Build history of the part. All positions in model axes, mm. A direction names the side the tool comes from. Give positions to 0.01 mm unless a question says otherwise; leave off trailing zeros. Loops run counter-clockwise (first coordinate to the right, second up) from the corner with the lowest first, then second, coordinate; pieces in that order, holes last. Notation, with made-up numbers: M 79,-9 L 126,-9 A30 cw 126,26 Z; hole C 19.5,50 d8. An arc over 180 degrees is marked long. Answer as a JSON object with one key per item and string values. Group by question number.
1. Slice it at D-D (z = 40). List the corners of the cut face in (x, y), then the cut area to 3 significant figures.
2. 3-axis set-ups, long thin cutter, end or side, ignore diameter. For faces 1 (the face through (25, 17.526, 25)), 2 (the face through (-44, 0, 0)), 3 (the face through (-43, 0, 17)): which of +Z, -Z, +X, -X, +Y, -Y reach the whole face in a straight line?
3. Slice it at C-C (x = 11.5). List the corners of the cut face in (y, z).
4. Slice it at B-B (x = 0). List the corners of the cut face in (y, z).
5. Mould opens along X. For faces 4 (the face through (35.708, 8.64, -35.446)), 5 (the face through (-1, -128.778, -1)), 6 (the face through (-57.095, 8.64, -2.513)) say: released by +X, released by -X, zero draft, split by the parting line, or undercut.
6. Slice it at A-A (z = 0). List the corners of the cut face in (x, y), then the cut area to 3 significant figures.
7. Drop flat-ended pins along their axis: pin 1 Ø7.5 at (x, z) = (46.101, 0) entering from +Y; pin 2 Ø6 at (y, z) = (-79.5, 35.5) entering from +X; pin 3 Ø10 at (x, y) = (8.5, -8) entering from -Z. Give the stop position or say it passes through.
8. Drill centre lines: line 1 along Z through (x, y) = (0, 12); line 2 along Y through (x, z) = (-22, 19); line 3 along Y through (x, z) = (23, 50). Where is each one in solid material? Low to high. Write a range as [from, to].
from build123d import *

# Parameters (mm, degrees)
SKETCH1_R           = 57.15
SKETCH1_R_2         = 30.099
EXTRUDE_THIN1_DEPTH = 17.526
SKETCH2_R           = 4.2164
CUT_EXTRUDE2_DEPTH  = 17.526
CIRPATTERN1_COUNT   = 8
SKETCH5_R           = 45.72
EXTRUDE1_DEPTH      = 128.778


with BuildPart() as part:
    # Sketch1 → Extrude-Thin1 (new body)
    with BuildSketch(Plane(origin=(0, 0, 0), x_dir=(1, 0, 0), z_dir=(0, 1, 0))):
        Circle(SKETCH1_R)
        Circle(SKETCH1_R_2, mode=Mode.SUBTRACT)
    extrude(amount=EXTRUDE_THIN1_DEPTH)

    # Sketch2 → Cut-Extrude2 (cut)
    with BuildSketch(Plane(origin=(0, 0, 0), x_dir=(1, 0, 0), z_dir=(0, 1, 0))):
        with Locations(Location((0, 46.101, 0), (0, 0, 270))):
            Circle(SKETCH2_R)
    cut_extrude2 = extrude(amount=CUT_EXTRUDE2_DEPTH, mode=Mode.SUBTRACT)

    # CirPattern1: Cut-Extrude2 ×8 about axis
    cirpattern1_axis = Axis((0, 0, 0), (0, 1, 0))
    for i in range(1, CIRPATTERN1_COUNT):
        add(cut_extrude2.rotate(cirpattern1_axis, i * 360 / CIRPATTERN1_COUNT), mode=Mode.SUBTRACT)

    # Sketch5 → Extrude1 (add)
    with BuildSketch(Plane.XZ):
        with Locations(Location((0, 0, 0), (0, 0, 95.242365855))):
            Circle(SKETCH5_R)
    extrude(amount=EXTRUDE1_DEPTH)


solid = part.part
Established:
{
 "1": {"outline": "M -40.82,0 L -22.14,0 L -22.14,-128.78 L 22.14,-128.78 L 22.14,0 L 40.82,0 L 40.82,17.53 L -40.82,17.53 Z", "area": "7,130 mm^2"},
 "2": {"face 1": "+Z, -Z, +X, -X, +Y", "face 2": "+Y", "face 3": "-Y"},
 "3": {"outline": "M -128.78,-44.25 L 0,-44.25 L 0,-55.98 L 17.53,-55.98 L 17.53,-27.82 L 0,-27.82 L 0,27.82 L 17.53,27.82 L 17.53,55.98 L 0,55.98 L 0,44.25 L -128.78,44.25 Z"},
 "4": {"outline": "M -128.78,-45.72 L 0,-45.72 L 0,-41.88 L 17.53,-41.88 L 17.53,-30.1 L 0,-30.1 L 0,30.1 L 17.53,30.1 L 17.53,41.88 L 0,41.88 L 0,45.72 L -128.78,45.72 Z; M 0,-57.15 L 17.53,-57.15 L 17.53,-50.32 L 0,-50.32 Z; M 0,50.32 L 17.53,50.32 L 17.53,57.15 L 0,57.15 Z"},
 "5": {"face 4": "undercut", "face 5": "zero draft", "face 6": "split by the parting line"},
 "6": {"outline": "M -57.15,0 L -50.32,0 L -50.32,17.53 L -57.15,17.53 Z; M -45.72,-128.78 L 45.72,-128.78 L 45.72,0 L 41.88,0 L 41.88,17.53 L 30.1,17.53 L 30.1,0 L -30.1,0 L -30.1,17.53 L -41.88,17.53 L -41.88,0 L -45.72,0 Z; M 50.32,0 L 57.15,0 L 57.15,17.53 L 50.32,17.53 Z", "area": "12,400 mm^2"},
 "7": {"pin 1": "stops at y = 0", "pin 2": "stops at x = 32.16", "pin 3": "stops at z = -45.59"},
 "8": {"line 1": "z = [-57.15, -50.32], [-41.88, -30.1], [30.1, 41.88], [50.32, 57.15]", "line 2": "y = [-128.78, 0]", "line 3": "y = [0, 17.53]"}
}
